The model under review builds one solid part; all positions refer to its coordinate system, in mm. A direction names the side the tool comes from. Give positions to 0.01 mm unless a question says otherwise; leave off trailing zeros. Loops run counter-clockwise (first coordinate to the right, second up) from the corner with the lowest first, then second, coordinate; pieces in that order, holes last. Notation, with made-up numbers: (85, 42) -> (140, 42) arc R15 ccw to (140, 51) -> close; hole circle Ø11 at (-30.75, 4.25). An arc over 180 degrees is marked (long way). Write each question's results on one line, items separated by ' | '. Start each with the question number.
Q1. We need section A-A (x = 0). Write out the cut boundary in (y, z), plus the area to 3 significant figures.
Q2. We need section C-C (y = 9). Write out the cut boundary in (x, z).
Q3. Mouldability with a two-part tool opening along Y and no side actions: class faces 1 (the face through (6.31, 1.23, -20.03)), 2 (the face through (22, 0, 0)), 3 (the face through (13.843, 3.362, 18.054)) as released by +Y, released by -Y, zero draft, split by the parting line, or undercut.
Q4. Machinability: for faces 4 (the face through (6.31, 10.26, -20.03)), 5 (the face through (20, 2.5, 7)), 6 (the face through (14, 20, -14)), which of the approach directions +Z, -Z, +X, -X, +Y, -Y give a long, thin tool a straight path to every point of the face, cutting with its end or side? Answer none if there is none.
Q5. Wall thickness on L1, parallel to X at y = 17.45, z = 0; L2, parallel to Y at x = -10.5, z = 19; L3, parallel to Z at x = -18.5, y = 5: over which ranges is each line inside the solid? List them lowest first. Write a range as [from, to].
Q6. Insertion check: pin 1 Ø4 at (x, y) = (29, 17.5) entering from -Z; pin 2 Ø8 at (x, y) = (-21.5, 3) entering from -Z; pin 3 Ø10 at (x, y) = (7.5, 7) entering from +Z. Each pin has a flat end and moves straight along its axis. Give the tip position at first contact, or say it passes through.
Q7. We need section B-B (z = 0). Write out the cut boundary in (x, y), plus the area to 3 significant figures.
from build123d import *

# Parameters (mm, degrees)
SKETCH_5_R          = 21
CUT_EXTRUDE_1_DEPTH = 16.5
SKETCH_6_W          = 1.75
SKETCH_6_H          = 1.7
SKETCH_7_R          = 17
CUT_EXTRUDE_2_DEPTH = 16


with BuildPart() as part:
    # 草图1 → 旋转1 (revolve)
    with BuildSketch(Plane.XY, mode=Mode.PRIVATE) as revolve_1_sk:
        with BuildLine():
            Line((10, 0), (33, 0))
            ThreePointArc((33, 0), (43, 10), (33, 20))
            Line((33, 20), (10, 20))
            Line((10, 20), (10, 0))
        make_face()
    revolve(revolve_1_sk.sketch.rotate(Axis((0, 0, 0), (0, 1, 0)), 90), axis=Axis((0, 0, 0), (0, 1, 0)))

    # 草图5 → 切除-拉伸1 (cut)
    with BuildSketch(Plane.XZ):
        with Locations(Location((0, 0, 0), (0, 0, 270))):
            Circle(SKETCH_5_R)
    extrude(amount=-CUT_EXTRUDE_1_DEPTH, mode=Mode.SUBTRACT)

    # 草图6 → 切除-旋转1 (revolve, cut)
    with BuildSketch(Plane(origin=(0, 0, 0), x_dir=(0, 0, -1), z_dir=(1, 0, 0))):
        with Locations((21.875, 3.35)):
            Rectangle(SKETCH_6_W, SKETCH_6_H)
    revolve(axis=Axis((0, 0, 0), (0, 1, 0)), mode=Mode.SUBTRACT)

    # 草图7 → 切除-拉伸2 (cut)
    with BuildSketch(Plane(origin=(0, 20, 0), x_dir=(1, 0, 0), z_dir=(0, 1, 0))):
        with Locations(Location((0, 0, 0), (0, 0, 270))):
            Circle(SKETCH_7_R)
    extrude(amount=-CUT_EXTRUDE_2_DEPTH, mode=Mode.SUBTRACT)


solid = part.part
Output:
1) outline: (0, -33) arc R10 ccw to (20, -33) -> (20, -17) -> (16.5, -17) -> (16.5, -21) -> (4.2, -21) -> (4.2, -22.75) -> (2.5, -22.75) -> (2.5, -21) -> (0, -21) -> close; (0, 21) -> (2.5, 21) -> (2.5, 22.75) -> (4.2, 22.75) -> (4.2, 21) -> (16.5, 21) -> (16.5, 17) -> (20, 17) -> (20, 33) arc R10 ccw to (0, 33) -> close | area: 816 mm2
2) outline: circle Ø85.9 at (0, 0); hole circle Ø42 at (0, 0)
3) face 1: zero draft | face 2: released by -Y | face 3: undercut
4) face 4: -Y | face 5: none | face 6: +Z, -Z, +X, -X, +Y
5) L1: [-39.67, -17], [17, 39.67] | L2: [0, 2.5], [4.2, 20] | L3: [-37.33, -9.94], [9.94, 37.33]
6) pin 1: z = -30.25 | pin 2: z = -37.72 | pin 3: z = 42.87
7) outline: (-33, 0) -> (-21, 0) -> (-21, 2.5) -> (-22.75, 2.5) -> (-22.75, 4.2) -> (-21, 4.2) -> (-21, 16.5) -> (-17, 16.5) -> (-17, 20) -> (-33, 20) arc R10 ccw to start; (17, 16.5) -> (21, 16.5) -> (21, 4.2) -> (22.75, 4.2) -> (22.75, 2.5) -> (21, 2.5) -> (21, 0) -> (33, 0) arc R10 ccw to (33, 20) -> (17, 20) -> close | area: 816 mm2
